Verification items for the finished model (mm, model axes). Face numbers are marked on the shaded views. A direction names the side the tool comes from. Coordinates: 2 decimals unless noted, no trailing zeros. Order: outer loops, then holes, each group sorted by start corner. A loop starts at its lowest first (then second) coordinate and runs counter-clockwise, first axis right, second up.
Q1. Set-up check for the marked faces 1 and 2: record each of +Z, -Z, +X, -X, +Y, -Y from which the full face is reachable in a straight line by a thin tool's end or side.
Q2. Depth check by flat-ended pin: P1, Ø8, axis at y = 98.5, z = 10.5, coming from the +X side; P2, Ø3, axis at x = 0, y = 27.5, coming from the -Z side; P3, Ø3, axis at x = -23.5, z = 6.5, coming from the +Y side (3 decimals); P4, Ø12, axis at x = 10, z = -8.5, coming from the -Y side. Enter the tip coordinate at first touch or a pass-through.
Q3. Thickness scan on line 1 (Y direction, x = 0, z = 19.5) (3 decimals); line 2 (Z direction, x = 0, y = 60); line 3 (X direction, y = 141.5, z = -12). Record the ranges inside material, lowest first.
Q4. Cross-section at C-C, the plane z = 9. Record the boundary of the cut face in (x, y) (3 decimals), and give its area (3 significant figures).
Q5. Cross-section at D-D, the plane x = -11. Record the boundary of the cut face in (y, z), and give its area (3 significant figures).
Q6. Draft check along Z on the marked faces 3, 4 and 5. Enter one of: pulls with the +Z half, pulls with the -Z half, needs draft (parallel to the pull), parting line crosses it, or undercut.
Q7. Cross-section at A-A, the plane x = 0. Record the boundary of the cut face in (y, z) (1 decimal), and give its area (3 significant figures).
Q8. Cross-section at B-B, the plane y = 65.5. Record the boundary of the cut face in (x, z) (1 decimal).
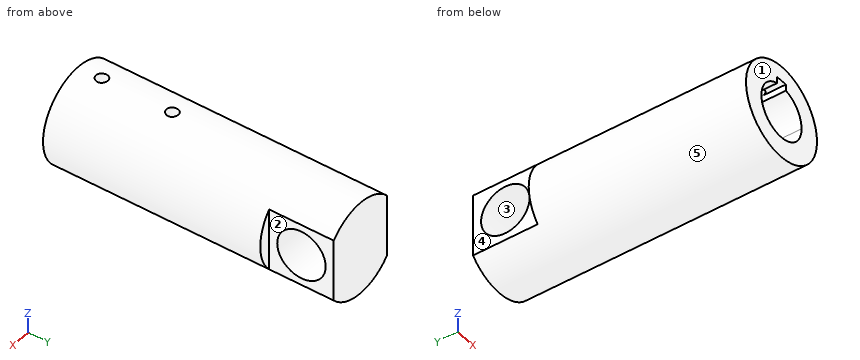
from build123d import *

# Parameters (mm, degrees)
F0_R     = 25.4
F1_DEPTH = 152.4
F3_DEPTH = 76.2
F5_DEPTH = 7.9375
F7_DEPTH = 34.925
F9_D     = 26.19502


with BuildPart() as f1:
    # F0 (on Front) → F1 (new body)
    with BuildSketch(Plane.XZ):
        Circle(F0_R)
    extrude(amount=-F1_DEPTH)

    # F2 (on face) → F3 (cut)
    with BuildSketch(Plane.XZ):
        with BuildLine():
            ThreePointArc((-3.175, 13.995376951), (-8.9550761024, -11.214179105), (14.351, 0))
            ThreePointArc((14.351, 0), (11.214179105, 8.9550761024), (3.175, 13.995376951))
            Line((3.175, 13.995376951), (3.175, 11.1125))
            Line((3.175, 11.1125), (-3.175, 11.1125))
            Line((-3.175, 11.1125), (-3.175, 13.995376951))
        make_face()
        with BuildLine():
            Line((3.175, 11.1125), (3.175, 13.995376951))
            ThreePointArc((3.175, 13.995376951), (0, 14.351), (-3.175, 13.995376951))
            Line((-3.175, 13.995376951), (-3.175, 11.1125))
            Line((-3.175, 11.1125), (3.175, 11.1125))
        make_face()
        with BuildLine():
            ThreePointArc((-3.175, 13.995376951), (0, 14.351), (3.175, 13.995376951))
            Line((3.175, 13.995376951), (3.175, 17.4625))
            Line((3.175, 17.4625), (-3.175, 17.4625))
            Line((-3.175, 17.4625), (-3.175, 13.995376951))
        make_face()
    extrude(amount=-F3_DEPTH, mode=Mode.SUBTRACT)

    # F4 (on face) → F5 (cut, through all)
    with BuildSketch(Plane(origin=(0, 0, 17.4625), x_dir=(1, 0, 0), z_dir=(0, 0, -1))):
        with BuildLine():
            ThreePointArc((-3.175, -12.7), (0, -15.875), (3.175, -12.7))
            ThreePointArc((3.175, -12.7), (0, -9.525), (-3.175, -12.7))
        make_face()
        with BuildLine():
            ThreePointArc((-3.175, -50.8), (0, -53.975), (3.175, -50.8))
            ThreePointArc((3.175, -50.8), (0, -47.625), (-3.175, -50.8))
        make_face()
    extrude(amount=-F5_DEPTH, mode=Mode.SUBTRACT)

    # F6 (on face) → F7 (cut)
    with BuildSketch(Plane(origin=(0, 152.4, 0), x_dir=(-1, 0, 0), z_dir=(0, 1, 0))):
        with BuildLine():
            Line((-19.05, -16.8005208253), (-19.05, 16.8005208253))
            ThreePointArc((-19.05, 16.8005208253), (-25.4, 0), (-19.05, -16.8005208253))
        make_face()
        with BuildLine():
            ThreePointArc((19.05, -16.8005208253), (23.759524406, -8.9802561211), (25.4, 0))
            ThreePointArc((25.4, 0), (23.759524406, 8.9802561211), (19.05, 16.8005208253))
            Line((19.05, 16.8005208253), (19.05, -16.8005208253))
        make_face()
    extrude(amount=-F7_DEPTH, mode=Mode.SUBTRACT)

    # F9 (through all)
    with Locations(Plane.YZ.offset(19.05)):
        with Locations((134.9375, 0)):
            Hole(F9_D / 2)


solid = f1.part
Check values:
1. face 1: +Z, -Z, +X, -X, -Y
1. face 2: +Z, -Z, +X, +Y
2. P1: stops at x = 24.55
2. P2: stops at z = -25.4
2. P3: stops at y = 117.475
2. P4: stops at y = 0
3. line 1: y = 0 to 9.525, 15.875 to 47.625, 53.975 to 152.4
3. line 2: z = -25.4 to -14.35, 17.46 to 25.4
3. line 3: x = -19.05 to 19.05
4. outline: (-23.752, 0) - (-11.178, 0) - (-11.178, 76.2) - (11.178, 76.2) - (11.178, 0) - (23.752, 0) - (23.752, 117.475) - (19.05, 117.475) - (19.05, 125.422) - (-19.05, 125.422) - (-19.05, 117.475) - (-23.752, 117.475) - close; (-19.05, 144.453) - (19.05, 144.453) - (19.05, 152.4) - (-19.05, 152.4) - close
4. area: 4,480 mm2
5. outline: (0, -22.89) - (152.4, -22.89) - (152.4, 22.89) - (0, 22.89) - (0, 9.22) - (76.2, 9.22) - (76.2, -9.22) - (0, -9.22) - close; hole circle Ø26.2 at (134.94, 0)
5. area: 5,030 mm2
6. face 3: undercut
6. face 4: needs draft
6. face 5: parting line crosses it
7. outline: (0, -25.4) - (152.4, -25.4) - (152.4, 25.4) - (54, 25.4) - (54, 17.5) - (76.2, 17.5) - (76.2, -14.4) - (0, -14.4) - close; (0, 17.5) - (9.5, 17.5) - (9.5, 25.4) - (0, 25.4) - close; (15.9, 17.5) - (47.6, 17.5) - (47.6, 25.4) - (15.9, 25.4) - close; hole circle Ø26.2 at (134.9, 0)
7. area: 4,680 mm2
8. outline: circle Ø50.8 at (0, 0); hole (-3.2, 14) arc R14.4 ccw (long way) to (3.2, 14) - (3.2, 17.5) - (-3.2, 17.5) - close
